from build123d import *

# Parameters (mm, degrees)
SKETCH1_W           = 886
SKETCH1_H           = 800
BOSS_EXTRUDE1_DEPTH = 866
SKETCH2_W           = 750
SKETCH2_H           = 830
CUT_EXTRUDE1_DEPTH  = 850
CUT_EXTRUDE2_DEPTH  = 288
BOSS_EXTRUDE2_DEPTH = 50
HOLE1_D             = 150
HOLE1_DEPTH         = 68


with BuildPart() as part:
    # Sketch1 → Boss-Extrude1 (new body)
    with BuildSketch(Plane.XY.offset(433)):
        with Locations((0, 382)):
            Rectangle(SKETCH1_W, SKETCH1_H)
    extrude(amount=-BOSS_EXTRUDE1_DEPTH)

    # Sketch2 → Cut-Extrude1 (cut)
    with BuildSketch(Plane(origin=(-425, 0, 0), x_dir=(0, -1, 0), z_dir=(-1, 0, 0))):
        with Locations((-382, 0)):
            Rectangle(SKETCH2_W, SKETCH2_H)
    extrude(amount=-CUT_EXTRUDE1_DEPTH, mode=Mode.SUBTRACT)

    # Sketch3 → Cut-Extrude2 (cut)
    with BuildSketch(Plane(origin=(0, 0, -433), x_dir=(-1, 0, 0), z_dir=(0, 0, -1))):
        with BuildLine():
            Line((-300, 725), (-300, 715))
            ThreePointArc((-300, 715), (-295.606601718, 704.393398282), (-285, 700))
            Line((-285, 700), (285, 700))
            ThreePointArc((285, 700), (295.606601718, 704.393398282), (300, 715))
            Line((300, 715), (300, 725))
            ThreePointArc((300, 725), (295.606601718, 735.606601718), (285, 740))
            Line((285, 740), (-285, 740))
            ThreePointArc((-285, 740), (-295.606601718, 735.606601718), (-300, 725))
        make_face()
    extrude(amount=-CUT_EXTRUDE2_DEPTH, mode=Mode.SUBTRACT)

    # Sketch4 → Boss-Extrude2 (add)
    with BuildSketch(Plane(origin=(0, 0, 415), x_dir=(-1, 0, 0), z_dir=(0, 0, -1))):
        with BuildLine():
            ThreePointArc((0, 80.419601085), (-175, 110), (0, 139.580398915))
            ThreePointArc((0, 139.580398915), (175, 110), (0, 80.419601085))
        make_face()
    extrude(amount=BOSS_EXTRUDE2_DEPTH)

    # Hole1
    with Locations(Plane(origin=(0, 0, 365), x_dir=(-1, 0, 0), z_dir=(0, 0, -1))):
        with Locations((-85, 110), (85, 110)):
            Hole(HOLE1_D / 2, depth=HOLE1_DEPTH)


solid = part.part
The model under review builds one solid part; all positions refer to its coordinate system, in mm. A direction names the side the tool comes from. Round coordinates to 2 decimals unless told otherwise and drop trailing zeros. Loops run counter-clockwise (first coordinate to the right, second up) from the corner with the lowest first, then second, coordinate; pieces in that order, holes last. Notation, with made-up numbers: M 8,55 L 55,55 A24 ccw 55,93 Z; hole C -3.5,80 d4. An arc over 180 degrees is marked long. Answer as CSV lines item,"result". Start each with the question number.
Item 1: For faces 1 (the face through (-174.93, 113.54, 390.35)), 2 (the face through (29.722, 160.689, 399.476)), 3 (the face through (443, 376, 6)), list the 3-axis set-ups (+Z, -Z, +X, -X, +Y, -Y) from which the entire face can be reached by the end or side of a thin tool; tool diameter is ignored.
Item 2: Consider section D-D (x = 321.5). Write out the cut boundary in (y, z).
Item 3: Insertion check: P1, Ø10, axis at x = -64.5, y = 116, coming from the +Z side. The pin has a flat end and moves straight along its axis. Give the tip position at first contact, or say it passes through.
Item 4: Consider section C-C (z = -99.5). Write out the cut boundary in (x, y).
Item 5: Consider section A-A (x = 85). Write out the cut boundary in (y, z).
Item 6: Mouldability with a two-part tool opening along Z and no side actions: class faces 4 (the face through (-6, 782, 6)), 5 (the face through (-6, 7, -6)), 6 (the face through (-6, 388, 433)) as released by +Z, released by -Z, zero draft, split by the parting line, or undercut.
Item 7: Wall thickness on line 1 (Y direction, x = 85, z = 405); line 2 (Y direction, x = 307, z = 253); line 3 (Z direction, x = -168.5, y = 501): over which ranges is each line inside the solid? List them lowest first. Write a range as [from, to].
Item 8: Consider section B-B (y = 110). Write out the cut boundary in (x, z).
Answer:
1,face 1,"none"
1,face 2,"+Z"
1,face 3,"+Z, -Z, +X, +Y, -Y"
2,outline,"M -18,-433 L 782,-433 L 782,433 L -18,433 Z; hole M 7,-415 L 757,-415 L 757,415 L 7,415 Z"
3,P1,"stops at z = -415"
4,outline,"M -443,-18 L 443,-18 L 443,782 L -443,782 Z; hole M -425,7 L 425,7 L 425,757 L -425,757 Z"
5,outline,"M -18,-433 L 700,-433 L 700,-415 L 7,-415 L 7,415 L 20,415 L 20,365 L 35,365 L 35,433 L -18,433 Z; M 185,365 L 200,365 L 200,415 L 757,415 L 757,-415 L 740,-415 L 740,-433 L 782,-433 L 782,433 L 185,433 Z"
6,face 4,"zero draft"
6,face 5,"undercut"
6,face 6,"released by +Z"
7,line 1,"y = [-18, 7], [20, 35], [185, 200], [757, 782]"
7,line 2,"y = [-18, 7], [757, 782]"
7,line 3,"z = [-433, -415], [415, 433]"
8,outline,"M -443,-433 L 443,-433 L 443,433 L 160,433 L 160,365 L 175,365 L 175,415 L 425,415 L 425,-415 L -425,-415 L -425,415 L -175,415 L -175,365 L -160,365 L -160,433 L -443,433 Z; M -10,365 L 10,365 L 10,433 L -10,433 Z"
